from build123d import *

# Parameters (mm, degrees)
CROQUIS1_W              = 48.3
CROQUIS1_H              = 25.8
SALIENTE_EXTRUIR1_DEPTH = 1.7
CROQUIS2_W              = 25.7
CROQUIS2_H              = 18.9
SALIENTE_EXTRUIR2_DEPTH = 0.7
CROQUIS3_W              = 17.8
CROQUIS3_H              = 15.8
SALIENTE_EXTRUIR3_DEPTH = 2.5
CROQUIS4_W              = 5.7
CROQUIS4_H              = 7.52
SALIENTE_EXTRUIR4_DEPTH = 2.4
REDONDEO1_R             = 1


with BuildPart() as part:
    # Croquis1 → Saliente-Extruir1 (new body)
    with BuildSketch(Plane(origin=(0, 0, 0), x_dir=(1, 0, 0), z_dir=(0, 1, 0))):
        Rectangle(CROQUIS1_W, CROQUIS1_H)
    extrude(amount=SALIENTE_EXTRUIR1_DEPTH)

    # Croquis2 → Saliente-Extruir2 (add)
    with BuildSketch(Plane(origin=(0, 1.7, 0), x_dir=(1, 0, 0), z_dir=(0, 1, 0))):
        with Locations((11.3, -0.45)):
            Rectangle(CROQUIS2_W, CROQUIS2_H)
    extrude(amount=SALIENTE_EXTRUIR2_DEPTH)

    # Croquis3 → Saliente-Extruir3 (add)
    with BuildSketch(Plane(origin=(0, 2.4, 0), x_dir=(1, 0, 0), z_dir=(0, 1, 0))):
        with Locations((8.9, -0.45)):
            Rectangle(CROQUIS3_W, CROQUIS3_H)
    extrude(amount=SALIENTE_EXTRUIR3_DEPTH)

    # Croquis4 → Saliente-Extruir4 (add)
    with BuildSketch(Plane(origin=(0, 1.7, 0), x_dir=(1, 0, 0), z_dir=(0, 1, 0))):
        with Locations((-23, 0.12)):
            Rectangle(CROQUIS4_W, CROQUIS4_H)
    extrude(amount=SALIENTE_EXTRUIR4_DEPTH)

    # Redondeo1
    redondeo1_edges = [part.edges().sort_by_distance(p)[0] for p in [
        (24.15, 0.85, 12.9),
        (-24.15, 0.85, 12.9),
        (-24.15, 0.85, -12.9),
        (24.15, 0.85, -12.9),
    ]]
    fillet(redondeo1_edges, radius=REDONDEO1_R)


solid = part.part
Could you check a few things on this model? Use its own coordinates, in mm. A direction names the side the tool comes from. Coordinates: 2 decimals unless noted, no trailing zeros. Loops run counter-clockwise (first coordinate to the right, second up) from the corner with the lowest first, then second, coordinate; pieces in that order, holes last. Notation, with made-up numbers: (67, 83) -> (91, 83) arc R19 ccw to (91, 101) -> close; hole circle Ø11 at (21, 34). An arc over 180 degrees is marked (long way). Answer in a Markdown table with one row per item.
(1) Imagine slicing it at A-A (y = 2.9). List the corners of the cut face in (x, z) for me, plus the area to 3 significant figures.
Results found:
| item | result |
|---|---|
| outline | (-25.85, -3.88) -> (-20.15, -3.88) -> (-20.15, 3.64) -> (-25.85, 3.64) -> close; (0, -7.45) -> (17.8, -7.45) -> (17.8, 8.35) -> (0, 8.35) -> close |
| area | 324 mm^2 |
(2) Thinking about a two-plate mould opening in X: for faces 1 (the face through (23.849, 0.862, -12.615)), 2 (the face through (-24.15, 1, 0)), 3 (the face through (0, 4, 1)), 4 (the face through (-25, 1.7, 0)), which applies, released by +X, released by -X, zero draft, split by the parting line, or undercut?
Results found:
| item | result |
|---|---|
| face 1 | released by +X |
| face 2 | released by -X |
| face 3 | undercut |
| face 4 | zero draft |
(3) For faces 5 (the face through (9, 4, -7.45)), 6 (the face through (-23, 3, 3.64)), 7 (the face through (9, 4, 8.35)), 8 (the face through (-23, 3, -3.88)), 9 (the face through (17.8, 4, 1)), which set-ups out of +Z, -Z, +X, -X, +Y, -Y let a thin tool reach every point of the face, with its end or its side?
Results found:
| item | result |
|---|---|
| face 5 | -Z, +X, -X, +Y |
| face 6 | +Z, -X, +Y |
| face 7 | +Z, +X, -X, +Y |
| face 8 | -Z, -X, +Y |
| face 9 | +Z, -Z, +X, +Y |
(4) Imagine slicing it at D-D (y = 0.55). List the corners of the cut face in (x, z) for me, plus the area to 3 significant figures.
Results found:
| item | result |
|---|---|
| outline | (-24.15, -11.9) arc R1 ccw to (-23.15, -12.9) -> (23.15, -12.9) arc R1 ccw to (24.15, -11.9) -> (24.15, 11.9) arc R1 ccw to (23.15, 12.9) -> (-23.15, 12.9) arc R1 ccw to (-24.15, 11.9) -> close |
| area | 1,250 mm^2 |
(5) Imagine slicing it at C-C (z = 1.25). List the corners of the cut face in (x, y) for me.
Results found:
| item | result |
|---|---|
| outline | (-25.85, 1.7) -> (-24.15, 1.7) -> (-24.15, 0) -> (24.15, 0) -> (24.15, 2.4) -> (17.8, 2.4) -> (17.8, 4.9) -> (0, 4.9) -> (0, 2.4) -> (-1.55, 2.4) -> (-1.55, 1.7) -> (-20.15, 1.7) -> (-20.15, 4.1) -> (-25.85, 4.1) -> close |
(6) Will these pins go through, and if not, where does the flat tip stop? pin 1 Ø2.5 at (x, y) = (-24, 3) entering from -Z; pin 2 Ø0.9 at (x, z) = (-25.5, -0.5) entering from -Y; pin 3 Ø2 at (x, y) = (5.5, 3.5) entering from +Z.
Results found:
| item | result |
|---|---|
| pin 1 | stops at z = -3.88 |
| pin 2 | stops at y = 1.7 |
| pin 3 | stops at z = 8.35 |
(7) If I drill on probe 1 along X at (y, z) = (0.2, -1.75); probe 2 along Y at (x, z) = (-17.5, -8.25); probe 3 along X at (y, z) = (2.15, -4.5), over which ranges is the centre line in solid material (lowest first)?
Results found:
| item | result |
|---|---|
| probe 1 | x = -24.15 to 24.15 |
| probe 2 | y = 0 to 1.7 |
| probe 3 | x = -1.55 to 24.15 |
(8) Imagine slicing it at B-B (x = 10). List the corners of the cut face in (y, z) for me, plus the area to 3 significant figures.
Results found:
| item | result |
|---|---|
| outline | (0, -12.9) -> (1.7, -12.9) -> (1.7, -9) -> (2.4, -9) -> (2.4, -7.45) -> (4.9, -7.45) -> (4.9, 8.35) -> (2.4, 8.35) -> (2.4, 9.9) -> (1.7, 9.9) -> (1.7, 12.9) -> (0, 12.9) -> close |
| area | 96.6 mm^2 |
